The model under review builds one solid part; all positions refer to its coordinate system, in mm. A direction names the side the tool comes from. Round coordinates to 2 decimals unless told otherwise and drop trailing zeros. Loops run counter-clockwise (first coordinate to the right, second up) from the corner with the lowest first, then second, coordinate; pieces in that order, holes last. Notation, with made-up numbers: (-23.75, 89.25) -> (26.25, 89.25) arc R22 ccw to (26.25, 123.25) -> close; hole circle Ø9 at (69.5, 85). An arc over 180 degrees is marked (long way). Return JSON: item names as keys, results as strings. Group by question number.
```python
from build123d import *

# Parameters (mm, degrees)
F0_R      = 30.1625
F0_R_2    = 25.4
F1_DEPTH  = 190.5
F3_W      = 63.5
F3_H      = 63.5
F3_R      = 12.7
F4_DEPTH  = 19.05
F6_W      = 63.5
F6_H      = 63.5
F7_DEPTH  = 19.05
F8_W      = 38.1
F8_H      = 25.4
F9_DEPTH  = 98.425
F10_W     = 38.1
F10_H     = 12.7
F13_D     = 12.7
F14_W     = 55.815736
F14_H     = 42.682048
F15_DEPTH = 9.525


with BuildPart() as f1:
    # F0 (on Top) → F1 (new body, symmetric)
    with BuildSketch(Plane.XY):
        Circle(F0_R)
        Circle(F0_R_2, mode=Mode.SUBTRACT)
    extrude(amount=F1_DEPTH, both=True)

    # F3 (on offset) → F4 (join)
    with BuildSketch(Plane.XY.offset(190.5)):
        Rectangle(F3_W, F3_H)
        Circle(F3_R, mode=Mode.SUBTRACT)
    extrude(amount=F4_DEPTH)

    # F6 (on offset) → F7 (join)
    with BuildSketch(Plane(origin=(0, 0, -190.5), x_dir=(1, 0, 0), z_dir=(0, 0, -1))):
        Rectangle(F6_W, F6_H)
    extrude(amount=F7_DEPTH)

    # F8 (on face) → F9 (join)
    with BuildSketch(Plane(origin=(0, 0, -209.55), x_dir=(1, 0, 0), z_dir=(0, 0, -1))):
        Rectangle(F8_W, F8_H)
    extrude(amount=F9_DEPTH)

    # F10 (on face) → F11 (revolve)
    with BuildSketch(Plane(origin=(0, 0, -307.975), x_dir=(1, 0, 0), z_dir=(0, 0, -1))):
        with Locations((0, 6.35)):
            Rectangle(F10_W, F10_H)
    revolve(axis=Axis((0, 0, -307.975), (1, 0, 0)))

    # F13 (through all)
    with Locations(Plane.YZ.offset(19.05)):
        with Locations((0, -307.975)):
            Hole(F13_D / 2)

    # F14 (on Right) → F15 (cut, symmetric)
    with BuildSketch(Plane.YZ):
        with Locations((-0.949135, -300.741024)):
            Rectangle(F14_W, F14_H)
    extrude(amount=F15_DEPTH, both=True, mode=Mode.SUBTRACT)


solid = f1.part
```
1. We need section B-B, the plane z = 116.5. Write out the cut boundary in (x, y) (1 decimal), then the cut area to 3 significant figures.
2. We need section D-D, the plane z = -248. Write out the cut boundary in (x, y).
3. For P1, Ø10, axis at y = -13, z = -232.5, coming from the +X side; P2, Ø9.5, axis at x = 0, y = 6, coming from the -Z side; P3, Ø11.5, axis at x = 6, z = -252.5, coming from the -Y side, all flat-tipped, find the tip position at first contact; note any pin that passes through.
4. We need section C-C, the plane y = 0. Give the number of separate pieces and of enclosed holes in the cut face, then the cut area to 3 significant figures.
5. Draft analysis for pull direction X (two halves, no side actions). For faces 4 (the face through (9.525, 0, -295)), 5 (the face through (-31.75, 0, -200)), 6 (the face through (-19, 24, 190.5)), 7 (the face through (-30.133, 1.326, 2.667)), state which applies: pulls with the +X half, pulls with the -X half, needs draft (parallel to the pull), parting line crosses it, or undercut.
6. Tool access review of faces 1 (the face through (0, -12.7, -247)), 2 (the face through (-19.05, 0, -264)), 3 (the face through (0, 0, -190.5)): name each direction out of +Z, -Z, +X, -X, +Y, -Y from which nothing blocks a thin tool from reaching the whole face with its end or side.
7. We need section A-A, the plane x = 0. Write out the cut boundary in (y, z), then the cut area to 3 significant figures.
8. Wall thickness on line 1 (Z direction, x = -1.5, y = -20.5); line 2 (Z direction, x = -12.5, y = 0) (3 decimals); line 3 (Y direction, x = -2, z = 2): over which ranges is each line inside the solid? List them lowest first.
Check sheet entries:
{
 "1": {"outline": "circle Ø60.3 at (0, 0); hole circle Ø50.8 at (0, 0)", "area": "831 mm²"},
 "2": {"outline": "(-19.05, -12.7) -> (19.05, -12.7) -> (19.05, 12.7) -> (-19.05, 12.7) -> close"},
 "3": {"P1": "stops at x = 19.05", "P2": "stops at z = -279.4", "P3": "stops at y = -12.7"},
 "4": {"separate pieces": "3", "enclosed holes": "0", "area": "8,770 mm²"},
 "5": {"face 4": "undercut", "face 5": "pulls with the -X half", "face 6": "needs draft", "face 7": "parting line crosses it"},
 "6": {"face 1": "-Z, +X, -X, -Y", "face 2": "-Z, -X, +Y, -Y", "face 3": "none"},
 "7": {"outline": "(-31.75, -209.55) -> (-12.7, -209.55) -> (-12.7, -279.4) -> (12.7, -279.4) -> (12.7, -209.55) -> (31.75, -209.55) -> (31.75, -190.5) -> (30.16, -190.5) -> (30.16, 190.5) -> (31.75, 190.5) -> (31.75, 209.55) -> (12.7, 209.55) -> (12.7, 190.5) -> (25.4, 190.5) -> (25.4, -190.5) -> (-25.4, -190.5) -> (-25.4, 190.5) -> (-12.7, 190.5) -> (-12.7, 209.55) -> (-31.75, 209.55) -> (-31.75, 190.5) -> (-30.16, 190.5) -> (-30.16, -190.5) -> (-31.75, -190.5) -> close", "area": "7,340 mm²"},
 "8": {"line 1": "z = -209.55 to -190.5, 190.5 to 209.55", "line 2": "z = -320.675 to -314.325, -301.625 to -190.5", "line 3": "y = -30.1 to -25.32, 25.32 to 30.1"}
}
